from build123d import *

# Parameters (mm, degrees)
F0_R      = 177.8
F1_DEPTH  = 101.6
F2_R      = 153.042574
F3_DEPTH  = 12.7
F4_R      = 153.04262
F5_DEPTH  = 12.7
F7_W      = 69.85
F7_H      = 50.8
F8_DEPTH  = 63.5
F10_W     = 12.7
F10_H     = 12.7
F11_DEPTH = 31.75
F12_W     = 6.35
F12_H     = 12.7
F13_DEPTH = 19.05
F14_W     = 6.35
F14_H     = 12.7
F15_DEPTH = 19.05


with BuildPart() as f1:
    # F0 (on Front) → F1 (new body)
    with BuildSketch(Plane.XZ):
        Circle(F0_R)
    extrude(amount=-F1_DEPTH)

    # F2 (on face) → F3 (cut)
    with BuildSketch(Plane(origin=(0, 101.6, 0), x_dir=(-1, 0, 0), z_dir=(0, 1, 0))):
        Circle(F2_R)
    extrude(amount=-F3_DEPTH, mode=Mode.SUBTRACT)

    # F4 (on face) → F5 (cut)
    with BuildSketch(Plane.XZ):
        Circle(F4_R)
    extrude(amount=-F5_DEPTH, mode=Mode.SUBTRACT)

    # F7 (on offset) → F8 (cut)
    with BuildSketch(Plane.YZ.offset(177.8)):
        with Locations((50.85966, -82.082137)):
            Rectangle(F7_W, F7_H)
    extrude(amount=-F8_DEPTH, mode=Mode.SUBTRACT)

    # F10 (on offset) → F11 (join)
    with BuildSketch(Plane.YZ.offset(114.3)):
        with Locations((51.032025, -82.255941)):
            Rectangle(F10_W, F10_H)
    extrude(amount=F11_DEPTH)

    # F12 (on face) → F13 (join)
    with BuildSketch(Plane.XZ.offset(-44.682025)):
        with Locations((142.875, -82.255941)):
            Rectangle(F12_W, F12_H)
    extrude(amount=F13_DEPTH)

    # F14 (on face) → F15 (join)
    with BuildSketch(Plane(origin=(0, 57.382025, 0), x_dir=(-1, 0, 0), z_dir=(0, 1, 0))):
        with Locations((-142.875, -82.255941)):
            Rectangle(F14_W, F14_H)
    extrude(amount=F15_DEPTH)


solid = f1.part
Can you work these out from the model? Positions are in its coordinate system, mm. A direction names the side the tool comes from. Coordinates: 2 decimals unless noted, no trailing zeros. Write each loop counter-clockwise with the first axis right and the second up, starting at its lowest first coordinate (ties: lowest second). Pieces come first, ordered by that corner, then holes. Notation, with made-up numbers: (18.5, -26) - (56.5, -26) arc R7 cw to (56.5, -21) - close; hole circle Ø4 at (-4, 77.5). An arc over 180 degrees is marked (long way). Return JSON: item names as keys, results as strings. Group by question number.
Item 1: We'd pull the mould along Z, two halves only. Please class faces 6 (the face through (142, 50, -56.682)), 7 (the face through (-131.046, 50.089, 120.166)), 8 (the face through (146.05, 51, -82)), 9 (the face through (2, 88.9, 2)): pulls with the +Z half, pulls with the -Z half, needs draft (parallel to the pull), parting line crosses it, or undercut.
Item 2: If we section it at A-A (y = 36.5): Write out the boundary of the cut face in (x, z).
Item 3: If we section it at B-B (z = 0): Write out the boundary of the cut face in (x, y), then the cut area to 3 significant figures.
Item 4: I'm going to push flat-ended pins straight in: pin 1 Ø5 at (x, y) = (15.5, 31.5) entering from -Z; pin 2 Ø12 at (x, y) = (122.5, 44) entering from +Z; pin 3 Ø13.5 at (x, y) = (122.5, 46.5) entering from +Z. Where does each tip first touch, or does it pass through?
Item 5: Please list where these lines run through material, in increasing order: probe 1 along Z at (x, y) = (0, 92); probe 2 along Y at (x, z) = (-50, -112.5); probe 3 along Z at (x, y) = (-99, 89.5).
Item 6: Which directions (+Z, -Z, +X, -X, +Y, -Y) give clear straight access to the entire face, cutting with the end or side of a thin tool? Please do faces 1 (the face through (134, 51, -75.906)), 2 (the face through (78, 0, 133)), 3 (the face through (139.7, 67, -82)), 4 (the face through (-145.975, 95.339, 45.97)), 5 (the face through (145.975, 6.261, 45.97)).
Item 7: If we section it at C-C (x = 100): Write out the boundary of the cut face in (y, z), then the cut area to 3 significant figures.
Return value:
{
 "1": {"face 6": "undercut", "face 7": "parting line crosses it", "face 8": "needs draft", "face 9": "undercut"},
 "2": {"outline": "(114.3, -107.48) - (114.3, -56.68) - (168.52, -56.68) arc R177.8 ccw (long way) to (141.63, -107.48) - close; (139.7, -88.61) - (146.05, -88.61) - (146.05, -75.91) - (139.7, -75.91) - close"},
 "3": {"outline": "(-177.8, 0) - (-153.04, 0) - (-153.04, 12.7) - (153.04, 12.7) - (153.04, 0) - (177.8, 0) - (177.8, 101.6) - (153.04, 101.6) - (153.04, 88.9) - (-153.04, 88.9) - (-153.04, 101.6) - (-177.8, 101.6) - close", "area": "28,400 mm^2"},
 "4": {"pin 1": "stops at z = -177.32", "pin 2": "stops at z = 134.32", "pin 3": "stops at z = 134.96"},
 "5": {"probe 1": "z = -177.8 to -153.04, 153.04 to 177.8", "probe 2": "y = 12.7 to 88.9", "probe 3": "z = -147.69 to -116.71, 116.71 to 147.69"},
 "6": {"face 1": "+X", "face 2": "+Z, -Z, +X, -X, -Y", "face 3": "none", "face 4": "+Y", "face 5": "-Y"},
 "7": {"outline": "(0, -147.01) - (101.6, -147.01) - (101.6, -115.85) - (88.9, -115.85) - (88.9, 115.85) - (101.6, 115.85) - (101.6, 147.01) - (0, 147.01) - (0, 115.85) - (12.7, 115.85) - (12.7, -115.85) - (0, -115.85) - close", "area": "24,000 mm^2"}
}
